```python
from build123d import *

# Parameters (mm, degrees)
BOSS_EXTRUDE1_DEPTH   = 10.16
F_4_CLEARANCE_HOLE1_D = 3.4544
SKETCH4_R             = 1.905
CUT_EXTRUDE1_DEPTH    = 8.62
CUT_EXTRUDE1_TAPER    = -20
SKETCH5_R             = 4.1275
CUT_EXTRUDE2_DEPTH    = 1.27
SKETCH6_W             = 25.4
SKETCH6_H             = 2.54
BOSS_EXTRUDE2_DEPTH   = 7.62
SKETCH7_R             = 5.08
PRINTTABS_DEPTH       = 0.4


with BuildPart() as part:
    # Sketch1 → Boss-Extrude1 (new body)
    with BuildSketch(Plane.XY):
        with BuildLine():
            Line((-17.145, -3.81), (17.145, -3.81))
            ThreePointArc((17.145, -3.81), (20.955, 0), (17.145, 3.81))
            Line((17.145, 3.81), (-17.145, 3.81))
            Line((-17.145, 3.81), (-17.145, -3.81))
        make_face()
    extrude(amount=BOSS_EXTRUDE1_DEPTH)

    # #4 Clearance Hole1 (through all)
    with Locations(Plane.XY.offset(10.16)):
        with Locations((17.145, 0)):
            Hole(F_4_CLEARANCE_HOLE1_D / 2)

    # Sketch4 → Cut-Extrude1 (cut, through all)
    with BuildSketch(Plane(origin=(0, -3.81, 0), x_dir=(1, 0, 0), z_dir=(0, 1, 0))):
        with Locations((-8.89, -5.08)):
            Circle(SKETCH4_R)
    extrude(amount=CUT_EXTRUDE1_DEPTH, taper=CUT_EXTRUDE1_TAPER, mode=Mode.SUBTRACT)

    # Sketch5 → Cut-Extrude2 (cut)
    with BuildSketch(Plane.XZ.offset(3.81)):
        with Locations((-8.89, 5.08)):
            Circle(SKETCH5_R)
    extrude(amount=-CUT_EXTRUDE2_DEPTH, mode=Mode.SUBTRACT)

    # Sketch6 → Boss-Extrude2 (add, through all)
    with BuildSketch(Plane.XZ.offset(3.81)):
        with Locations((-4.445, 11.43)):
            Rectangle(SKETCH6_W, SKETCH6_H)
        with Locations((-4.445, -1.27)):
            Rectangle(SKETCH6_W, SKETCH6_H)
    extrude(amount=-BOSS_EXTRUDE2_DEPTH)

    # Sketch7 → PrintTabs (add)
    with BuildSketch(Plane(origin=(0, 3.81, 0), x_dir=(1, 0, 0), z_dir=(0, 1, 0))):
        with Locations((8.255, 2.54)):
            Circle(SKETCH7_R)
        with Locations((-17.145, -12.7)):
            Circle(SKETCH7_R)
        with Locations((-17.145, 2.54)):
            Circle(SKETCH7_R)
        with Locations((8.255, -10.16)):
            Circle(SKETCH7_R)
        with Locations((17.145, -5.08)):
            Circle(SKETCH7_R)
    extrude(amount=-PRINTTABS_DEPTH)


solid = part.part
```
Here's how the part is built. I have some questions about the finished solid (model axes, mm). A direction names the side the tool comes from. Coordinates: 2 decimals unless noted, no trailing zeros. Loops run counter-clockwise (first coordinate to the right, second up) from the corner with the lowest first, then second, coordinate; pieces in that order, holes last. Notation, with made-up numbers: M 48,-17.75 L 107,-17.75 A11 ccw 107,-12.75 Z; hole C 65.5,6.25 d8. An arc over 180 degrees is marked long. One line per item, written item: value.
1. Imagine slicing it at D-D (z = 4). State how many separate pieces and enclosed holes the cut face has, and give its area (3 significant figures).
Geometry says:
separate pieces: 2
enclosed holes: 1
area: 224 mm2
2. Please list where these lines run through material, in increasing order: probe 1 along Z at (x, y) = (-8.89, -3.5); probe 2 along X at (y, z) = (1, 3.5) (3 decimals); probe 3 along Z at (x, y) = (11, -1.5).
Geometry says:
probe 1: z = -2.54 to 0.95, 9.21 to 12.7
probe 2: x = -17.145 to -12.187, -5.593 to 15.737, 18.553 to 20.821
probe 3: z = 0 to 10.16
3. Thinking about a two-plate mould opening in Z: for faces 6 (the conical face through (-11.912, -0.732, 4.947)), 7 (the flat face through (-5, 0, -2.54)), 8 (the flat face through (0, -3.81, 5)), which applies, +Z half, -Z half, draft (parallel to the pull), parting line (faces both ways), or undercut?
Geometry says:
face 6: undercut
face 7: -Z half
face 8: draft
4. Imagine slicing it at C-C (z = 14.5). List the corners of the cut face in (x, y) for me.
Geometry says:
outline: M -21.9,3.41 L -12.39,3.41 L -12.39,3.81 L -21.9,3.81 Z; M 5.61,3.41 L 10.9,3.41 L 10.9,3.81 L 5.61,3.81 Z
5. On a 3-axis mill with a long thin cutter (end or side, diameter ignored), from which of +Z, -Z, +X, -X, +Y, -Y can I reach the whole of each face in a straight line? I mean faces 1 (the flat face through (15, 0, 10.16)), 2 (the flat face through (0, 3.81, 5)), 3 (the flat face through (-7, -2.54, 3)), 4 (the cylindrical face through (9.48, 3.61, 15.09)), 5 (the flat face through (8.255, 0, -1)). Say none if no direction works.
Geometry says:
face 1: +Z, +X, -Y
face 2: +Z, -Z, +X, -X, +Y
face 3: -Y
face 4: +Z, +Y, -Y
face 5: -Z, +X, -Y
6. Imagine slicing it at A-A (y = 0). List the corners of the cut face in (x, z) for me (3 decimals).
Geometry says:
outline: M -17.145,-2.54 L 8.255,-2.54 L 8.255,0 L 15.418,0 L 15.418,10.16 L 8.255,10.16 L 8.255,12.7 L -17.145,12.7 Z; M 18.872,0 L 20.955,0 L 20.955,10.16 L 18.872,10.16 Z; hole C -8.89,5.08 d6.583
7. Will these pins go through, and if not, where does the flat tip stop? pin 1 Ø3 at (y, z) = (1.5, 11.5) entering from +X; pin 2 Ø4 at (x, y) = (-8, 1) entering from +Z; pin 3 Ø2 at (x, y) = (-4, 0.5) entering from -Z.
Geometry says:
pin 1: stops at x = 20.86
pin 2: stops at z = 12.7
pin 3: stops at z = -2.54
8. Imagine slicing it at B-B (x = -8.89). List the corners of the cut face in (y, z) for me.
Geometry says:
outline: M -3.81,-2.54 L 3.81,-2.54 L 3.81,0.4 L -2.54,2.71 L -2.54,0.95 L -3.81,0.95 Z; M -3.81,9.21 L -2.54,9.21 L -2.54,7.45 L 3.81,9.76 L 3.81,12.7 L -3.81,12.7 Z
